```python
from build123d import *

# Parameters (mm, degrees)
CROQUIS1_R                                           = 42.5
SALIENTE_EXTRUIR1_DEPTH                              = 2.5
REFRENTADO_PARA_TORNILLO_CON_CABEZA_TRON_D           = 3.4
REFRENTADO_PARA_TORNILLO_CON_CABEZA_TRON_CBORE_D     = 7
REFRENTADO_PARA_TORNILLO_CON_CABEZA_TRON_CBORE_DEPTH = 2.4
TALADRO_DE_MARGEN_PARA_M41_D                         = 4.5
CORTAR_EXTRUIR1_REACH                                = 62.312


with BuildPart() as part:
    # Croquis1 → Saliente-Extruir1 (new, symmetric)
    with BuildSketch(Plane.XY):
        Circle(CROQUIS1_R)
    extrude(amount=SALIENTE_EXTRUIR1_DEPTH, both=True)

    # Refrentado para tornillo con cabeza troncocónica de M31 (through all)
    with Locations(Plane.XY.offset(2.5)):
        with Locations((0, 27.75), (24.032204955, -13.875), (-24.032204955, -13.875)):
            CounterBoreHole(REFRENTADO_PARA_TORNILLO_CON_CABEZA_TRON_D / 2, REFRENTADO_PARA_TORNILLO_CON_CABEZA_TRON_CBORE_D / 2, REFRENTADO_PARA_TORNILLO_CON_CABEZA_TRON_CBORE_DEPTH)

    # Taladro de margen para M41 (through all)
    with Locations(Plane.XY.offset(2.5)):
        with Locations((0, -27), (-23.382685902, 13.5), (23.382685902, 13.5)):
            Hole(TALADRO_DE_MARGEN_PARA_M41_D / 2)

    # Croquis8 → Cortar-Extruir1 (cut, up to next)
    with BuildSketch(Plane.XY.offset(2.5), mode=Mode.PRIVATE) as cortar_extruir1_sk1:
        Polygon((-14.820508076, 14.330127019), (0, 5.773502692), (14.820508076, 14.330127019), (19.820508076, 5.669872981), (5, -2.886751346), (5, -20), (-5, -20), (-5, -2.886751346), (-19.820508076, 5.669872981), align=None)
    cortar_extruir1_tool1 = extrude(cortar_extruir1_sk1.sketch, amount=-CORTAR_EXTRUIR1_REACH, mode=Mode.PRIVATE) & part.part
    add(cortar_extruir1_tool1.solids().sort_by_distance((0, 0, 2.5))[0], mode=Mode.SUBTRACT)


solid = part.part
```
Model file for the job. Use its own axes, mm. A direction names the side the tool comes from. Round coordinates to 2 decimals unless told otherwise and drop trailing zeros. Write each loop counter-clockwise with the first axis right and the second up, starting at its lowest first coordinate (ties: lowest second). Pieces come first, ordered by that corner, then holes. Notation, with made-up numbers: M 29,25 L 66,25 A13 ccw 66,50 Z; hole C -14.5,19 d3. An arc over 180 degrees is marked long. Put each result on its own line as item: value.
Item 1: Probe L1, parallel to Y at x = 0, z = 0.95; L2, parallel to Y at x = 0, z = -0.35; L3, parallel to X at y = 9, z = 1.05. List the from-to ranges inside material, lowest first. Write a range as from..to.
Responses:
L1: -42.5..-29.25, -24.75..-20, 5.77..24.25, 31.25..42.5
L2: -42.5..-29.25, -24.75..-20, 5.77..26.05, 29.45..42.5
L3: -41.54..-17.9, -5.59..5.59, 17.9..41.54
Item 2: Cut at C-C (z = -1.7). State how many separate pieces and enclosed holes the cut face has, and give its area (3 significant figures).
Responses:
separate pieces: 1
enclosed holes: 7
area: 5,040 mm²
Item 3: Cut at B-B (x = -12). List the corners of the cut face in (y, z), and give its area (3 significant figures).
Responses:
outline: M -40.77,-2.5 L 1.15,-2.5 L 1.15,2.5 L -40.77,2.5 Z; M 12.7,-2.5 L 40.77,-2.5 L 40.77,2.5 L 12.7,2.5 Z
area: 350 mm²
Item 4: Cut at A-A (y = 0). List the corners of the cut face in (x, z).
Responses:
outline: M -42.5,-2.5 L -10,-2.5 L -10,2.5 L -42.5,2.5 Z; M 10,-2.5 L 42.5,-2.5 L 42.5,2.5 L 10,2.5 Z
Item 5: Flat gauge pins, fed straight in: P1, Ø4.5, axis at x = 24.03, y = -13.88, coming from the +Z side; P2, Ø1, axis at y = -8.5, z = 0.5, coming from the +X side; P3, Ø1, axis at x = 0.5, z = -2, coming from the -Y side. Where does each tip first touch, or does it go through?
Responses:
P1: z = 0.1
P2: x = 41.74
P3: y = -42.5
Item 6: Cut at D-D (y = 27.75). List the corners of the cut face in (x, z).
Responses:
outline: M -32.19,-2.5 L -1.7,-2.5 L -1.7,0.1 L -3.5,0.1 L -3.5,2.5 L -32.19,2.5 Z; M 1.7,-2.5 L 32.19,-2.5 L 32.19,2.5 L 3.5,2.5 L 3.5,0.1 L 1.7,0.1 Z
Item 7: Tool access for faces 4 (the flat face through (5, -11, 0)), 5 (the flat face through (-26, -15, 0.1)), 6 (the flat face through (-1, 10, 2.5)): list every direction of +Z, -Z, +X, -X, +Y, -Y with a clear straight run to the whole face (end or side of a thin tool).
Responses:
face 4: +Z, -Z
face 5: +Z
face 6: +Z, +X, -X, +Y, -Y
Item 8: Mould opens along X. For faces 1 (the cylindrical face through (-33.727, -25.861, 0.035)), 2 (the flat face through (-1, 10, -2.5)), 3 (the cylindrical face through (23.248, -15.383, -1.218)) say: +X half, -X half, draft (parallel to the pull), parting line (faces both ways), or undercut.
Responses:
face 1: parting line
face 2: draft
face 3: undercut
